Part model, mm, in its own coordinate system. Coordinates: 2 decimals unless noted, no trailing zeros. Loops run counter-clockwise (first coordinate to the right, second up) from the corner with the lowest first, then second, coordinate; pieces in that order, holes last. Notation, with made-up numbers: (66, 3) - (92, 3) arc R27 ccw to (92, 42) - close; hole circle Ø10 at (53, 10). An arc over 180 degrees is marked (long way). Answer as CSV lines item,"result".
from build123d import *

# Parameters (mm, degrees)
PAD003_DEPTH = 1.5
FILLET011_R  = 0.5
SKETCH023_W  = 6
SKETCH023_H  = 1
PAD004_DEPTH = 0.1


with BuildPart() as part:
    # Sketch020 → Pad003 (new body)
    with BuildSketch(Plane.XZ):
        with BuildLine():
            Line((-6.125, 1.875), (-6.125, -1.875))
            ThreePointArc((-4.875, -3.125), (-5.758883, -2.758883), (-6.125, -1.875))
            Line((-4.875, -3.125), (4.875, -3.125))
            ThreePointArc((6.125, -1.875), (5.758883, -2.758883), (4.875, -3.125))
            Line((6.125, -1.875), (6.125, 1.875))
            ThreePointArc((4.875, 3.125), (5.758883, 2.758883), (6.125, 1.875))
            Line((4.875, 3.125), (-4.875, 3.125))
            ThreePointArc((-6.125, 1.875), (-5.758883, 2.758883), (-4.875, 3.125))
        make_face()
    extrude(amount=PAD003_DEPTH)

    # Fillet011
    fillet011_edges = [part.edges().sort_by_distance(p)[0] for p in [
        (0, 0, -3.125),
    ]]
    fillet(fillet011_edges, radius=FILLET011_R)

    # Sketch023 (on Face4 of Fillet011) → Pad004 (join)
    with BuildSketch(Plane.XZ.offset(1.5)):
        Rectangle(SKETCH023_W, SKETCH023_H)
    extrude(amount=PAD004_DEPTH)


solid = part.part
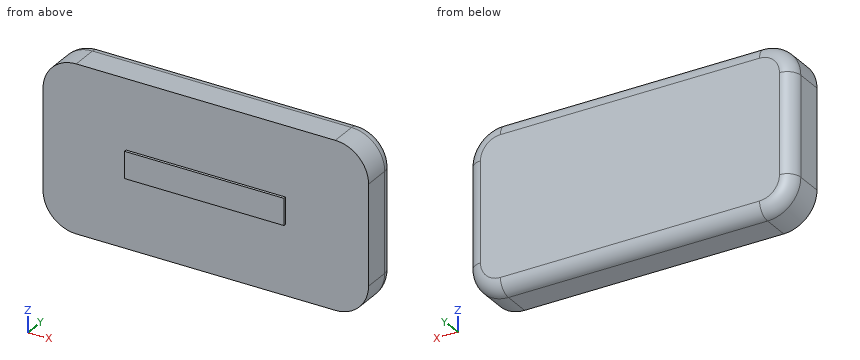
Q1. Saw through at A-A (x = -2.5). Give the cut face in (y, z) (3 decimals).
Results:
outline,"(-1.6, -0.5) - (-1.5, -0.5) - (-1.5, -3.125) - (-0.5, -3.125) arc R0.5 ccw to (0, -2.625) - (0, 2.625) arc R0.5 ccw to (-0.5, 3.125) - (-1.5, 3.125) - (-1.5, 0.5) - (-1.6, 0.5) - close"
Q2. Wall check: L1, parallel to Y at x = 3.5, z = -2.25; L2, parallel to X at y = -0.45, z = 1; L3, parallel to Z at x = 5.25, y = -1.05. Give the ranges that are in metal, low to high.
Results:
L1,"y = -1.5 to 0"
L2,"x = -6.12 to 6.12"
L3,"z = -3.07 to 3.07"
Q3. Saw through at C-C (z = -1.5). Give the cut face in (x, y) (3 decimals), then the cut area to 3 significant figures.
Results:
outline,"(-6.125, -1.5) - (6.125, -1.5) - (6.125, -0.5) arc R0.5 ccw to (5.625, 0) - (-5.625, 0) arc R0.5 ccw to (-6.125, -0.5) - close"
area,"18.3 mm^2"
Q4. Saw through at D-D (y = -0.15). Give the cut face in (x, z) (3 decimals).
Results:
outline,"(-5.982, -1.875) arc R1.107 ccw to (-4.875, -2.982) - (4.875, -2.982) arc R1.107 ccw to (5.982, -1.875) - (5.982, 1.875) arc R1.107 ccw to (4.875, 2.982) - (-4.875, 2.982) arc R1.107 ccw to (-5.982, 1.875) - close"
Q5. Saw through at B-B (y = -1.3). Give the cut face in (x, z) (3 decimals).
Results:
outline,"(-6.125, -1.875) arc R1.25 ccw to (-4.875, -3.125) - (4.875, -3.125) arc R1.25 ccw to (6.125, -1.875) - (6.125, 1.875) arc R1.25 ccw to (4.875, 3.125) - (-4.875, 3.125) arc R1.25 ccw to (-6.125, 1.875) - close"
